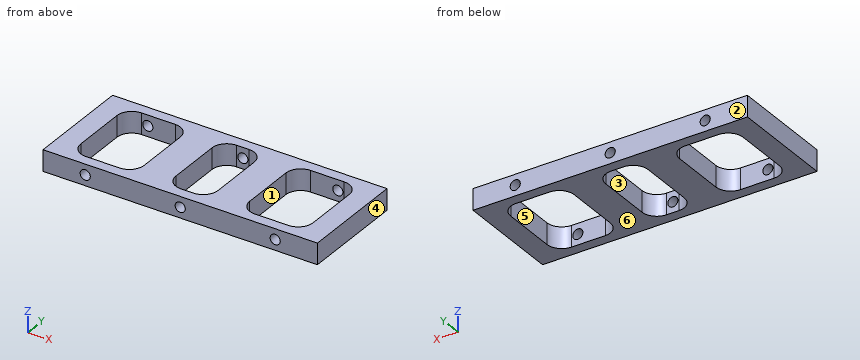
```python
from build123d import *

# Parameters (mm, degrees)
ESQUISSE1_W             = 130
ESQUISSE1_H             = 50
ESQUISSE1_W_2           = 110
ESQUISSE1_H_2           = 40
ESQUISSE1_W_3           = 15
BOSS_EXTRU_1_DEPTH      = 10
ESQUISSE2_R             = 2.4
ENL_V_MAT_EXTRU_1_DEPTH = 140.642400438
CONG_1_R                = 7


with BuildPart() as part:
    # Esquisse1 → Boss.-Extru.1 (new body)
    # profile 1 of 3: a face of its own
    with BuildSketch(Plane.XY):
        with Locations((65, 25)):
            Rectangle(ESQUISSE1_W, ESQUISSE1_H)
        with Locations((65, 25)):
            Rectangle(ESQUISSE1_W_2, ESQUISSE1_H_2, mode=Mode.SUBTRACT)
    # profile 2 of 3: a face of its own
    with BuildSketch(Plane.XY):
        with Locations((47.5, 25)):
            Rectangle(ESQUISSE1_W_3, ESQUISSE1_H_2)
    # profile 3 of 3: a face of its own
    with BuildSketch(Plane.XY):
        with Locations((82.5, 25)):
            Rectangle(ESQUISSE1_W_3, ESQUISSE1_H_2)
    extrude(amount=BOSS_EXTRU_1_DEPTH)

    # Esquisse2 → Enlèv. mat.-Extru.1 (cut, through all)
    with BuildSketch(Plane(origin=(0, 50, 0), x_dir=(1, 0, 0), z_dir=(0, 1, 0))):
        with Locations(Location((20, -5, 0), (0, 0, 270))):
            Circle(ESQUISSE2_R)
        with Locations(Location((65, -5, 0), (0, 0, 270))):
            Circle(ESQUISSE2_R)
        with Locations(Location((110, -5, 0), (0, 0, 270))):
            Circle(ESQUISSE2_R)
    extrude(amount=-ENL_V_MAT_EXTRU_1_DEPTH, mode=Mode.SUBTRACT)

    # Congé1
    cong_1_edges = [part.edges().sort_by_distance(p)[0] for p in [
        (40, 45, 5),
        (10, 45, 5),
        (10, 5, 5),
        (40, 5, 5),
        (120, 5, 5),
        (120, 45, 5),
        (90, 45, 5),
        (90, 5, 5),
        (75, 5, 5),
        (75, 45, 5),
        (55, 45, 5),
        (55, 5, 5),
    ]]
    fillet(cong_1_edges, radius=CONG_1_R)


solid = part.part
```
Model file for the job. Use its own axes, mm. Face numbers are marked on the shaded views. A direction names the side the tool comes from. Coordinates: 2 decimals unless noted, no trailing zeros. Loops run counter-clockwise (first coordinate to the right, second up) from the corner with the lowest first, then second, coordinate; pieces in that order, holes last. Notation, with made-up numbers: (76.5, -20) - (108.5, -20) arc R21 ccw to (108.5, -10) - close; hole circle Ø5 at (51.25, -40). An arc over 180 degrees is marked (long way). Answer as a JSON object with one key per item and string values. Group by question number.
(1) Two-plate mould, pull along X, no slides. Class the marked faces 3, 4, 5 and 6: released by +X, released by -X, zero draft, split by the parting line, or undercut.
(2) Cut at C-C (y = 29). Give the cut face in (x, z).
(3) Cut at A-A (x = 20). Give the cut face in (y, z), then the cut area to 3 significant figures.
(4) Flat gauge pin, fed straight in: pin 1 (6 mm diameter, centred on x = 20, z = 5, fed in from +Y). Where does the tip first touch, or does it go through?
(5) Cut at D-D (x = 101). Give the cut face in (y, z), then the cut area to 3 significant figures.
(6) Tool access for the marked faces 1 and 2: list every direction of +Z, -Z, +X, -X, +Y, -Y with a clear straight run to the whole face (end or side of a thin tool).
(7) Cut at B-B (z = 8.75). Give the cut face in (x, y).
(8) Probe line 1 along X through (y, z) = (2.35, 5); line 2 along X through (y, z) = (32, 6.5); line 3 along Y through (x, z) = (17, 8.5). List the from-to ranges inside material, lowest first.
Geometry says:
{
 "1": {"face 3": "undercut", "face 4": "released by +X", "face 5": "undercut", "face 6": "zero draft"},
 "2": {"outline": "(0, 0) - (10, 0) - (10, 10) - (0, 10) - close; (40, 0) - (55, 0) - (55, 10) - (40, 10) - close; (75, 0) - (90, 0) - (90, 10) - (75, 10) - close; (120, 0) - (130, 0) - (130, 10) - (120, 10) - close"},
 "3": {"outline": "(0, 0) - (5, 0) - (5, 2.6) - (0, 2.6) - close; (0, 7.4) - (5, 7.4) - (5, 10) - (0, 10) - close; (45, 0) - (50, 0) - (50, 2.6) - (45, 2.6) - close; (45, 7.4) - (50, 7.4) - (50, 10) - (45, 10) - close", "area": "52.0 mm^2"},
 "4": {"pin 1": "stops at y = 50"},
 "5": {"outline": "(0, 0) - (5, 0) - (5, 10) - (0, 10) - close; (45, 0) - (50, 0) - (50, 10) - (45, 10) - close", "area": "100 mm^2"},
 "6": {"face 1": "+Z, -Z", "face 2": "+Z, -Z, +X, -X, +Y"},
 "7": {"outline": "(0, 0) - (130, 0) - (130, 50) - (0, 50) - close; hole (10, 12) arc R7 ccw to (17, 5) - (33, 5) arc R7 ccw to (40, 12) - (40, 38) arc R7 ccw to (33, 45) - (17, 45) arc R7 ccw to (10, 38) - close; hole (55, 12) arc R7 ccw to (62, 5) - (68, 5) arc R7 ccw to (75, 12) - (75, 38) arc R7 ccw to (68, 45) - (62, 45) arc R7 ccw to (55, 38) - close; hole (90, 12) arc R7 ccw to (97, 5) - (113, 5) arc R7 ccw to (120, 12) - (120, 38) arc R7 ccw to (113, 45) - (97, 45) arc R7 ccw to (90, 38) - close"},
 "8": {"line 1": "x = 0 to 17.6, 22.4 to 62.6, 67.4 to 107.6, 112.4 to 130", "line 2": "x = 0 to 10, 40 to 55, 75 to 90, 120 to 130", "line 3": "y = 0 to 5, 45 to 50"}
}
